Autodesk Inventor part; units mm, degrees
ref_plane "YZ Plane" through (0, 0, 0) normal (1, 0, 0) x (0, 1, 0)
ref_plane "XZ Plane" through (0, 0, 0) normal (0, 1, 0) x (-1, 0, 0)
ref_plane "XY Plane" through (0, 0, 0) normal (0, 0, 1) x (1, 0, 0)
sketch "Sketch1" plane through (0, 0, 0) normal (0, 0, 1) x (1, 0, 0)
  line L0 (-16.9, -16.9) -> (-16.9, 16.9)
  line L1 (-16.9, 16.9) -> (16.9, 16.9)
  line L2 (16.9, 16.9) -> (16.9, -16.9)
  line L3 (16.9, -16.9) -> (-16.9, -16.9)
  circle A0 centre (-20, 20) radius 2.75
  circle A1 centre (20, -20) radius 2.75
  circle A2 centre (20, 20) radius 2.75
  circle A3 centre (-20, -20) radius 2.75
  line L4 (-22.9, 22.9) -> (22.9, 22.9)
  line L5 (-22.9, -22.9) -> (-22.9, 22.9)
  line L6 (22.9, -22.9) -> (-22.9, -22.9)
  line L7 (22.9, 22.9) -> (22.9, -22.9)
  line L8 (23.9, 23.9) -> (-23.9, 23.9)
  line L9 (-23.9, 23.9) -> (-23.9, -23.9)
  line L10 (-23.9, -23.9) -> (23.9, -23.9)
  line L11 (23.9, -23.9) -> (23.9, 23.9)
  point P0 (0, 0)
  point P1 (0, 0)
  dimension "d8" = 1
extrude "Extrusion1" add sketch "Sketch1" along normal blind 4 contours A0 | A1 | A2 | A3 | L4 L7 L6 L5 | L11 L10 L9 L8
sketch "Sketch2" plane through (0, 0, 4) normal (0, 0, 1) x (1, 0, 0)
  line L0 (-16.9, 16.9) -> (16.9, 16.9)
  line L1 (16.9, 16.9) -> (16.9, -16.9)
  line L2 (16.9, -16.9) -> (-16.9, -16.9)
  line L3 (-16.9, -16.9) -> (-16.9, 16.9)
  line L4 (-16.9, -16.9) -> (-16.9, 16.9)
  line L5 (-16.9, 16.9) -> (16.9, 16.9)
  line L6 (16.9, 16.9) -> (16.9, -16.9)
  line L7 (16.9, -16.9) -> (-16.9, -16.9)
  circle A0 centre (-20, 20) radius 2.15
  circle A1 centre (20, -20) radius 2.15
  circle A2 centre (20, 20) radius 2.15
  circle A3 centre (-20, -20) radius 2.15
  line L8 (-22.9, 22.9) -> (22.9, 22.9)
  line L9 (-22.9, -22.9) -> (-22.9, 22.9)
  line L10 (22.9, -22.9) -> (-22.9, -22.9)
  line L11 (22.9, 22.9) -> (22.9, -22.9)
  point P0 (0, 0)
  point P1 (0, 0)
  dimension "d2" = 4.3
  dimension "d3" = 4.3
  dimension "d4" = 4.3
  dimension "d5" = 4.3
extrude "Extrusion2" cut sketch "Sketch2" against normal through all contours A0 | A1 | A2 | A3
ref_plane "Work Plane1" through (-20, -20, 4) normal (0, -1, 0) x (1, 0, 0)
sketch "Sketch3" plane through (-20, -20, 4) normal (0, -1, 0) x (1, 0, 0)
  line L0 (2.15, -4) -> (-2.15, -4)
  line L1 (-2.15, 0) -> (2.15, 0)
  line L2 (43.9, -4) -> (-3.9, -4)
  line L3 (-3.9, -4) -> (-3.9, 0)
  line L4 (43.9, 0) -> (-3.9, 0)
  line L5 (43.9, -4) -> (43.9, 0)
  line L6 (0, 2.9614) -> (0, -7.6552) construction
  arc A0 (-2.15, 0) -> (0, -4.1992) centre (0, -1.5492) ccw
  line L7 (0, 1.1008) -> (0, -4.1992)
  arc A1 (0, 1.1008) -> (-2.15, 0) centre (0, -1.5492) ccw
  arc A2 (0, -4.1992) -> (0, 1.1008) centre (0, -1.5492) ccw
  point P0 (20, -4)
  point P1 (0, -4)
  dimension "d10" = 5.3
revolve "Revolution1" cut sketch "Sketch3" angle 360 about axis through (-20, -20, 5.1008) along (0, 0, -1) contours A2 L7 L0 | L0 L7 L1 A2 | L1 L7 A2
pattern_linear "Rectangular Pattern1" count 2 spacing 40 along (1, 0, 0) count 2 spacing 40 along (0, 1, 0) of "Revolution1"
sketch "Sketch4" plane through (0, 0, 4) normal (0, 0, 1) x (1, 0, 0)
  circle A0 centre (20, 20) radius 2.15
  circle A1 centre (-20, 20) radius 2.15
  circle A2 centre (20, -20) radius 2.15
  circle A3 centre (-20, -20) radius 2.15
  line L0 (-16.9, 16.9) -> (16.9, 16.9)
  line L1 (16.9, 16.9) -> (16.9, -16.9)
  line L2 (16.9, -16.9) -> (-16.9, -16.9)
  line L3 (-16.9, -16.9) -> (-16.9, 16.9)
  line L4 (23.9, 23.9) -> (-23.9, 23.9)
  line L5 (-23.9, 23.9) -> (-23.9, -23.9)
  line L6 (-23.9, -23.9) -> (23.9, -23.9)
  line L7 (23.9, -23.9) -> (23.9, 23.9)
  line L8 (-33.46, 0) -> (33.46, 0) construction
  line L9 (0, -33.46) -> (0, 33.46) construction
  line L10 (-15, 23.9) -> (15, 23.9)
  line L11 (15, 23.9) -> (15, 16.9)
  line L12 (15, 16.9) -> (-15, 16.9)
  line L13 (-15, 16.9) -> (-15, 23.9)
  line L14 (-23.9, -15) -> (-23.9, 15)
  line L15 (-16.9, -15) -> (-23.9, -15)
  line L16 (-16.9, 15) -> (-16.9, -15)
  line L17 (-23.9, 15) -> (-16.9, 15)
  line L18 (15, -23.9) -> (-15, -23.9)
  line L19 (15, -16.9) -> (15, -23.9)
  line L20 (-15, -16.9) -> (15, -16.9)
  line L21 (-15, -23.9) -> (-15, -16.9)
  line L22 (23.9, 15) -> (23.9, -15)
  line L23 (16.9, 15) -> (23.9, 15)
  line L24 (16.9, -15) -> (16.9, 15)
  line L25 (23.9, -15) -> (16.9, -15)
  point P0 (0, 0)
  dimension "d18" = 30
  dimension "d21" = 360
extrude "Extrusion3" cut sketch "Sketch4" against normal blind 0.3 contours L13 L4 L11 L0 | L3 L15 L5 L17 | L23 L7 L25 L1 | L2 L19 L6 L21
sketch "Sketch5" plane through (-23.9, 23.9, 0) normal (0, 1, 0) x (1, 0, 0)
  line L0 (38.9, -3.7) -> (38.9, -4) construction
  line L1 (47.8, -4) -> (38.9, -4) construction
  line L2 (47.8, 0) -> (47.8, -4) construction
  line L3 (47.8, 0) -> (0, 0) construction
  line L4 (0, 0) -> (0, -4) construction
  line L5 (8.9, -4) -> (0, -4) construction
  line L6 (8.9, -4) -> (8.9, -3.7) construction
  line L7 (8.9, -3.7) -> (38.9, -3.7) construction
  line L8 (23.9, 0) -> (23.9, -19.2449) construction
  line L9 (38.9, -3.7) -> (8.9, -3.7)
  line L10 (8.9, -3.7) -> (23.9, -9.5) construction
  line L11 (23.9, -9.5) -> (38.9, -3.7) construction
  spline S0 degree 2 poles (8.9, -3.7) (23.9, -9.5) (38.9, -3.7) knots 1 1 1 2 2 2
  line L12 (23.9, -3.7) -> (23.9, -6.6) construction
  line L13 (9.225, -3.0751) -> (8.9, -3.7)
  line L14 (38.9, -4) -> (38.9, -3.7)
  line L15 (38.575, -3.0751) -> (38.9, -3.7)
  spline S1 degree 5 poles (9.225, -3.0751) (12.0305, -4.1545) (14.9217, -5.0099) (17.888, -5.6036) (23.9, -6.1963) (29.912, -5.6036) (32.8783, -5.0099) (35.7695, -4.1545) (38.575, -3.0751) knots 0 0 0 0 0 0 0.5 0.5 0.5 1 1 1 1 1 1
  dimension "d26" = 0.7
  dimension "d25" = 2.9
extrude "Extrusion4" add sketch "Sketch5" against normal up to surface (7 mm away) contours S0 L9 S1 | L9 S1 L15 | L13 S1 L9
sketch "Sketch6" plane through (-23.9, -23.9, 0) normal (0, -1, 0) x (1, 0, 0)
  line L0 (36.8497, 3.7) -> (10.9503, 3.7)
  spline S0 degree 5 poles (10.9504, 3.7) (13.4491, 4.5486) (16.01, 5.2141) (18.6221, 5.6716) (23.9, 6.1284) (29.1779, 5.6716) (31.79, 5.2141) (34.3509, 4.5486) (36.8496, 3.7) knots 0 0 0 0 0 0 0.5 0.5 0.5 1 1 1 1 1 1
  spline S1 degree 2 poles (38.9, 3.7) (23.9, 9.5) (8.9, 3.7) knots 0 0 0 1 1 1
  line L1 (8.9, 3.7) -> (8.9, 4)
  line L2 (7, 4) -> (8.9, 4)
  line L3 (7, 0) -> (7, 4)
  line L4 (40.8, 0) -> (7, 0)
  line L5 (40.8, 0) -> (40.8, 4)
  line L6 (38.9, 4) -> (40.8, 4)
  line L7 (38.9, 4) -> (38.9, 3.7)
  point P0 (23.9, 0)
extrude "Extrusion5" add sketch "Sketch6" against normal up to surface (7 mm away)
equation "\"d3\" = d2"
equation "\"d4\" = d2"
equation "\"d5\" = d2"
properties part number "30_Sampleclamp_generic"
Part model, mm, in its own coordinate system. A direction names the side the tool comes from. Coordinates: 2 decimals unless noted, no trailing zeros. Loops run counter-clockwise (first coordinate to the right, second up) from the corner with the lowest first, then second, coordinate; pieces in that order, holes last. Notation, with made-up numbers: M -36,13 L -2,13 A16 cw -2,41 Z; hole C 62.25,13.25 d7. An arc over 180 degrees is marked long. Use a Markdown table: item, result. Add a question column.
Q1. Cut at D-D (z = 2). Write the cut outline in (x, y).
Q2. Cut at C-C (y = 20). Give the number of separate pieces and of enclosed holes in the cut face, and give its area (3 significant figures).
Q3. Which spindle directions (+Z, -Z, +X, -X, +Y, -Y) get a long thin tool onto all of the face, cutting with end or side? Do faces 1 (the flat face through (0, 20, 3.7)), 2 (the flat face through (-16.9, 0, 2)), 3 (the flat face through (-19.5, 17.5, 4)), 4 (the flat face through (17, 20, 4)). Say none if no direction does.
Q4. Probe L1, parallel to Y at x = -20, z = 0.3; L2, parallel to Y at x = 7, z = 1.75. List the from-to ranges inside material, lowest first.
Q5. Cut at B-B (x = 20). Write the cut outline in (y, z).
Q6. Cut at A-A (y = 1.5). Write the cut outline in (x, z), and give its area (3 significant figures).
Q7. Pin check, flat tips, straight feed: P1, Ø2.5, axis at x = -20, y = -18, coming from the +Z side; P2, Ø2, axis at x = -19, y = -1, coming from the +Z side; P3, Ø2.5, axis at x = -20, y = 20, coming from the -Z side. Stop position of each tip, or through.
Q8. Mould opens along Z. For faces 5 (the flat face through (18, -18, 4)), 6 (the flat face through (0, -23.9, 3)), 7 (the flat face through (0, -20, 3.7)) say: +Z half, -Z half, draft (parallel to the pull), parting line (faces both ways), or undercut.
Worked out:
| question | item | result |
|---|---|---|
| 1 | outline | M -23.9,-23.9 L 23.9,-23.9 L 23.9,23.9 L -23.9,23.9 Z; hole C -20,-20 d5.22; hole C -20,20 d5.22; hole M -16.9,-16.9 L 16.9,-16.9 L 16.9,16.9 L -16.9,16.9 Z; hole C 20,-20 d5.22; hole C 20,20 d5.22 |
| 2 | separate pieces | 3 |
| 2 | enclosed holes | 1 |
| 2 | area | 164 mm2 |
| 3 | face 1 | +Y, -Y |
| 3 | face 2 | +Z, -Z |
| 3 | face 3 | +Z, -X, +Y, -Y |
| 3 | face 4 | +Z, +X, +Y, -Y |
| 4 | L1 | y = -23.9 to -22.15, -17.85 to 17.85, 22.15 to 23.9 |
| 4 | L2 | y = -23.9 to -16.9, 16.9 to 23.9 |
| 5 | outline | M -23.9,0 L -22.15,0 L -22.15,0.9 A2.65 cw -22.15,4 L -23.9,4 Z; M -17.85,0 L 17.85,0 L 17.85,0.9 A2.65 cw 17.85,4 L 15,4 L 15,3.7 L -15,3.7 L -15,4 L -17.85,4 A2.65 cw -17.85,0.9 Z; M 22.15,0 L 23.9,0 L 23.9,4 L 22.15,4 A2.65 cw 22.15,0.9 Z |
| 6 | outline | M -23.9,0 L -16.9,0 L -16.9,3.7 L -23.9,3.7 Z; M 16.9,0 L 23.9,0 L 23.9,3.7 L 16.9,3.7 Z |
| 6 | area | 51.8 mm2 |
| 7 | P1 | stops at z = 4 |
| 7 | P2 | stops at z = 3.7 |
| 7 | P3 | passes through |
| 8 | face 5 | +Z half |
| 8 | face 6 | draft |
| 8 | face 7 | undercut |
